Could you check a few things on this drawing? It's one solid part, dimensions in mm from its lowest x, y, z. A direction names the side the tool comes from. Coordinates: 2 decimals unless noted, no trailing zeros. Order: outer loops, then holes, each group sorted by start corner. A loop starts at its lowest first (then second) coordinate and runs counter-clockwise, first axis right, second up.
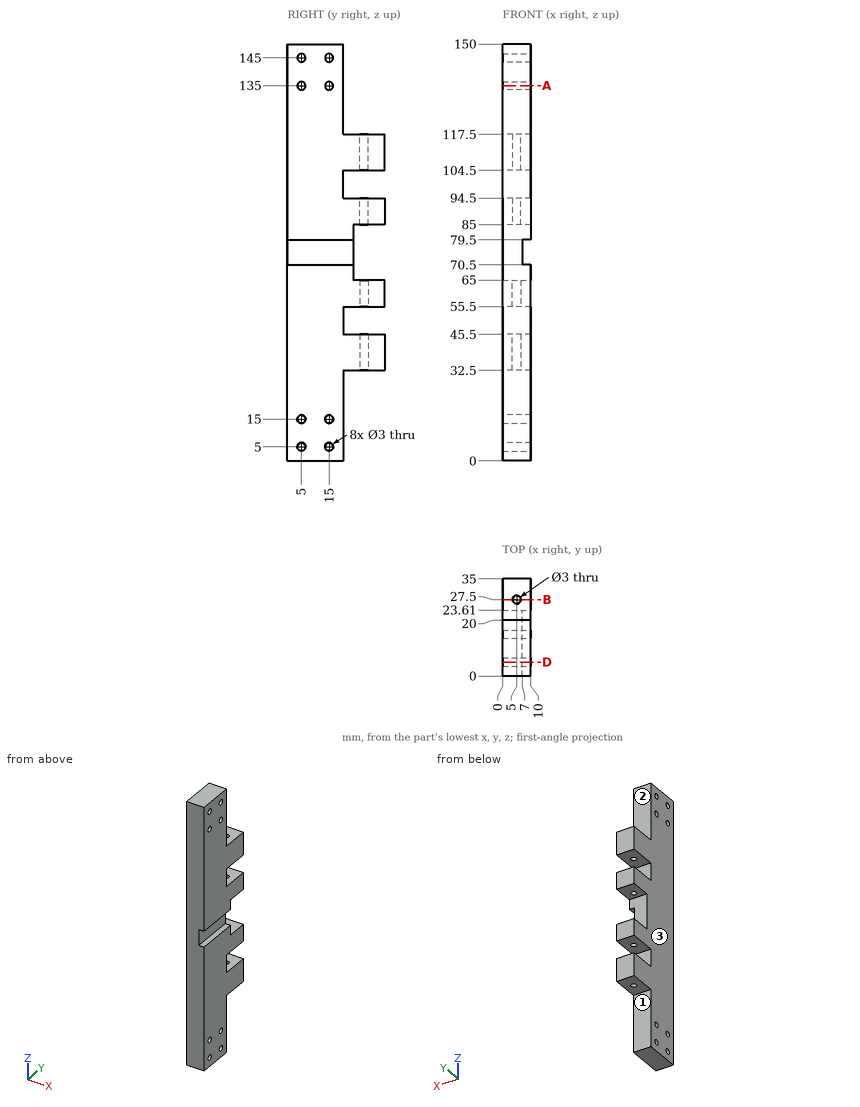
Item 1: For pin 1 Ø3 at (x, y) = (3.5, 30) entering from -Z; pin 2 Ø4 at (y, z) = (5, 15) entering from -X; pin 3 Ø5 at (x, z) = (5.5, 79) entering from +Y; pin 4 Ø5 at (x, y) = (5, 24) entering from +Z, each with a flat end and sliding along its axis, tell me the tip position at first contact or that it passes through.
Item 2: I need wall thicknesses on line 1 (Z direction, x = 7.5, y = 21); line 2 (Y direction, x = 3.5, z = 5); line 3 (Z direction, x = 2.5, y = 22). Which ranges of each line are inside material? Lowest first, please.
Item 3: Which directions (+Z, -Z, +X, -X, +Y, -Y) give clear straight access to the entire face, cutting with the end or side of a thin tool? Please do the marked faces 1, 2 and 3.
Item 4: Suppose I cut it at D-D (y = 5). List the corners of the cut face in (x, z) for me, and give its area (3 significant figures).
Item 5: Suppose I cut it at A-A (z = 135). List the corners of the cut face in (x, y) for me, and give its area (3 significant figures).
Item 6: Suppose I cut it at B-B (y = 27.5). Count the separate pieces of the cut face and the enclosed holes in it, and give its area (3 significant figures).
Geometry results:
1. pin 1: stops at z = 32.5
1. pin 2: stops at x = 0
1. pin 3: stops at y = 23.61
1. pin 4: stops at z = 117.5
2. line 1: z = 32.5 to 45.5, 55.5 to 70.5, 79.5 to 94.5, 104.5 to 117.5
2. line 2: y = 0 to 3.5, 6.5 to 13.5, 16.5 to 20
2. line 3: z = 32.5 to 45.5, 55.5 to 94.5, 104.5 to 117.5
3. face 1: -Z, +X, -X, +Y
3. face 2: +Z, +X, -X, +Y
3. face 3: +Z, -Z, -X, +Y, -Y
4. outline: (0, 0) - (10, 0) - (10, 3.5) - (0, 3.5) - close; (0, 6.5) - (10, 6.5) - (10, 13.5) - (0, 13.5) - close; (0, 16.5) - (10, 16.5) - (10, 70.5) - (7, 70.5) - (7, 79.5) - (10, 79.5) - (10, 133.5) - (0, 133.5) - close; (0, 136.5) - (10, 136.5) - (10, 143.5) - (0, 143.5) - close; (0, 146.5) - (10, 146.5) - (10, 150) - (0, 150) - close
4. area: 1,350 mm2
5. outline: (0, 0) - (10, 0) - (10, 3.5) - (0, 3.5) - close; (0, 6.5) - (10, 6.5) - (10, 13.5) - (0, 13.5) - close; (0, 16.5) - (10, 16.5) - (10, 20) - (0, 20) - close
5. area: 140 mm2
6. separate pieces: 8
6. enclosed holes: 0
6. area: 315 mm2
